```python
from build123d import *

# Parameters (mm, degrees)
F1_DEPTH = 63.5
F0_W     = 25.4
F0_H     = 19.05
F2_DEPTH = 25.4
F3_DEPTH = 7.9375
F5_R     = 6.35


with BuildPart() as f1:
    # F0 (on Front) → F1 (new body, symmetric)
    with BuildSketch(Plane.XZ):
        Polygon((22.225, 9.525), (-41.275, 9.525), (-41.275, -9.525), (41.275, -9.525), (41.275, 9.525), align=None)
    extrude(amount=F1_DEPTH, both=True)

    # F0 (on Front) → F2 (join, symmetric)
    with BuildSketch(Plane.XZ):
        with BuildLine():
            Line((22.225, 27.0002), (22.225, 9.525))
            Line((22.225, 9.525), (41.275, 9.525))
            Line((41.275, 9.525), (41.275, 27.0002))
            ThreePointArc((41.275, 27.0002), (45.9246798487, 38.2255201513), (57.15, 42.8752))
            Line((57.15, 42.8752), (60.325, 42.8752))
            Line((60.325, 42.8752), (60.325, 61.9252))
            Line((60.325, 61.9252), (57.15, 61.9252))
            ThreePointArc((57.15, 61.9252), (57.0455916297, 61.9250439351), (56.9411841925, 61.9245757419))
            ThreePointArc((56.9411841925, 61.9245757419), (32.3805781549, 51.6219661117), (22.225, 27.0002))
        make_face()
        with Locations((73.025, 52.4002)):
            Rectangle(F0_W, F0_H)
    extrude(amount=F2_DEPTH, both=True)

    # F0 (on Front) → F3 (join, symmetric)
    with BuildSketch(Plane.XZ):
        with BuildLine():
            add(Edge.make_bspline(
                [(-41.275, 9.525), (-41.1011968465, 50.1983393078), (21.0140626071, 61.7950971069), (56.9411841925, 61.9245757419)],
                knots=[0, 0, 0, 0, 111.2886193757, 111.2886193757, 111.2886193757, 111.2886193757], degree=3))
            Line((-41.275, 9.525), (22.225, 9.525))
            Line((22.225, 9.525), (22.225, 27.0002))
            ThreePointArc((22.225, 27.0002), (32.3805781549, 51.6219661117), (56.9411841925, 61.9245757419))
        make_face()
    extrude(amount=F3_DEPTH, both=True)

    # F0 (on Front) → F4 (revolve)
    with BuildSketch(Plane.XZ):
        Polygon((85.725, 66.675), (85.725, 61.9252), (85.725, 42.8752), (85.725, 38.1), (111.125, 38.1), (111.125, 66.675), align=None)
    revolve(axis=Axis((85.725, 0, 54.7751), (0, 0, 1)))

    # F5
    f5_edges = [f1.edges().sort_by_distance(p)[0] for p in [
        (41.275, -63.5, 0),
        (-41.275, -63.5, 0),
        (-41.275, 63.5, 0),
        (41.275, 63.5, 0),
    ]]
    fillet(f5_edges, radius=F5_R)


solid = f1.part
```
CAD build for the part. Positions are in the model's coordinates, mm. A direction names the side the tool comes from. Give positions to 0.01 mm unless a question says otherwise; leave off trailing zeros. Order: outer loops, then holes, each group sorted by start corner. A loop starts at its lowest first (then second) coordinate and runs counter-clockwise, first axis right, second up.
(1) Tool access for faces 5 (the flat face through (-2, 7.938, 30)), 6 (the flat face through (1, -36, 9.525)), 7 (the flat face through (46, -25.4, 42)), 8 (the flat face through (60, -2, 61.925)), 9 (the flat face through (86, 0, 38.1)): list every direction of +Z, -Z, +X, -X, +Y, -Y with a clear straight run to the whole face (end or side of a thin tool).
(2) Saw through at C-C, the plane y = -22.5. Give the cut face in (x, z) (3 decimals), then the cut area to 3 significant figures.
(3) Mould opens along X. For faces 1 (the flat face through (22.225, 17, 18)), 2 (the flat face through (46, 25.4, 42)), 3 (the cylindrical face through (39.464, -61.59, 0.133)), 4 (the flat face through (60, 2, 42.875)) say: released by +X, released by -X, zero draft, split by the parting line, or undercut.
(4) Drill centre lines: L1, parallel to Y at x = -24, z = 37.5; L2, parallel to Z at x = -34, y = 19 (3 decimals); L3, parallel to X at y = 20, z = -3 (3 decimals). Where is each one in solid material? Low to high.
(5) Saw through at A-A, the plane x = 74.5. Give the cut face in (y, z) (3 decimals).
(6) Saw through at D-D, the plane y = 31.5. Give the cut face in (x, z) (3 decimals), then the cut area to 3 significant figures.
(7) Flat gauge pins, fed straight in: pin 1 (4 mm diameter, centred on x = 50.5, y = 8, fed in from -Z); pin 2 (3 mm diameter, centred on x = -15.5, y = 7.5, fed in from +Z); pin 3 (3 mm diameter, centred on x = -20.5, z = 27.5, fed in from -Y). Where does each tip first touch, or does it go through?
Results found:
1. face 5: +Z, -X, +Y
1. face 6: +Z, -X, -Y
1. face 7: +Z, +X, -X, -Y
1. face 8: +Z, -X
1. face 9: -Z, +X, +Y, -Y
2. outline: (-41.275, -9.525) - (41.275, -9.525) - (41.275, 27) arc R15.875 cw to (57.15, 42.875) - (73.939, 42.875) - (73.939, 38.1) - (97.511, 38.1) - (97.511, 66.675) - (73.939, 66.675) - (73.939, 61.925) - (57.15, 61.925) arc R34.925 ccw to (56.941, 61.925) arc R34.925 ccw to (22.225, 27) - (22.225, 9.525) - (-41.275, 9.525) - close
2. area: 3,660 mm2
3. face 1: released by -X
3. face 2: zero draft
3. face 3: released by +X
3. face 4: undercut
4. L1: y = -7.94 to 7.94
4. L2: z = -9.525 to 9.525
4. L3: x = -41.275 to 41.275
5. outline: (-25.4, 42.875) - (-22.785, 42.875) - (-22.785, 38.1) - (22.785, 38.1) - (22.785, 42.875) - (25.4, 42.875) - (25.4, 61.925) - (22.785, 61.925) - (22.785, 66.675) - (-22.785, 66.675) - (-22.785, 61.925) - (-25.4, 61.925) - close
6. outline: (-41.275, -9.525) - (41.275, -9.525) - (41.275, 9.525) - (-41.275, 9.525) - close
6. area: 1,570 mm2
7. pin 1: stops at z = 40.31
7. pin 2: stops at z = 47.11
7. pin 3: stops at y = -7.94
